Can you work these out from the model? Positions are in its coordinate system, mm. Face numbers are marked on the shaded views. Coordinates: 2 decimals unless noted, no trailing zeros. Write each loop counter-clockwise with the first axis right and the second up, starting at its lowest first coordinate (ties: lowest second). Pieces come first, ordered by that corner, then holes. Notation, with made-up numbers: (62, 71.5) -> (100, 71.5) arc R12 cw to (100, 80.5) -> close; hole circle Ø7 at (4, -26.75). An arc over 180 degrees is marked (long way). Use one line per item in the form item = value.
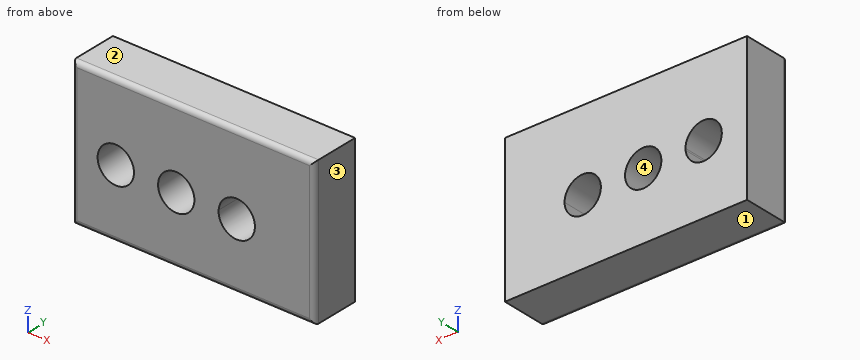
```python
from build123d import *

# Parameters (mm, degrees)
F0_W     = 254
F0_H     = 152.4
F1_DEPTH = 50.8
F3_DEPTH = 123.19
F4_R     = 5.08


with BuildPart() as f1:
    # F0 (on Front) → F1 (new body)
    with BuildSketch(Plane.XZ):
        with Locations((30.619834, 5.991532)):
            Rectangle(F0_W, F0_H)
    extrude(amount=F1_DEPTH)

    # F2 (on face) → F3 (cut)
    with BuildSketch(Plane.XZ.offset(50.8)):
        with BuildLine():
            ThreePointArc((-6.468596, 0), (12.581404, -19.05), (31.631404, 0))
            ThreePointArc((31.631404, 0), (12.581404, 19.05), (-6.468596, 0))
        make_face()
        with BuildLine():
            ThreePointArc((-31.782277, 1.811433), (-69.860685, 2.718177), (-31.868596, 0))
            ThreePointArc((-31.868596, 0), (-31.803869, 0.904689), (-31.782277, 1.811433))
        make_face()
        with BuildLine():
            ThreePointArc((95.098651, -1.116608), (76.607195, 17.925202), (57.031404, 0))
            ThreePointArc((57.031404, 0), (75.490107, -20.158418), (95.098651, -1.116608))
        make_face()
    extrude(amount=-F3_DEPTH, mode=Mode.SUBTRACT)

    # F4
    f4_edges = [f1.edges().sort_by_distance(p)[0] for p in [
        (30.619834, -50.8, -70.208468),
        (157.619834, -50.8, 5.991532),
        (30.619834, -50.8, 82.191532),
        (-96.380166, -50.8, 5.991532),
    ]]
    fillet(f4_edges, radius=F4_R)


solid = f1.part
```
Q1. Suppose I cut it at A-A (y = -35). Write out the boundary of the cut face in (x, z).
Return value:
outline = (-96.38, -70.21) -> (157.62, -70.21) -> (157.62, 82.19) -> (-96.38, 82.19) -> close; hole (-31.87, 0) arc R19.05 ccw to (-31.78, 1.81) arc R19.05 ccw (long way) to start; hole circle Ø38.1 at (12.58, 0); hole circle Ø38.1 at (76.05, -1.12)
Q2. If I drill on line 1 (X direction, y = -46, z = 13.5); line 2 (Z direction, x = 69, y = -15); line 3 (X direction, y = -46, z = -32), over which ranges is the centre line in solid material (lowest first)? Write a range as from..to.
Return value:
line_1 = -96.37..-65.87, -35.79..-0.86, 26.02..63.83, 88.27..157.61
line_2 = -70.21..-18.81, 16.58..82.19
line_3 = -96.37..157.61
Q3. Thinking about a two-plate mould opening in Z: for the marked faces 1, 2, 3 and 4, which applies, released by +Z, released by -Z, zero draft, split by the parting line, or undercut?
Return value:
face_1 = released by -Z
face_2 = released by +Z
face_3 = zero draft
face_4 = undercut
Q4. Suppose I cut it at D-D (x = 86). Write out the boundary of the cut face in (y, z).
Return value:
outline = (-50.8, -65.13) arc R5.08 ccw to (-45.72, -70.21) -> (0, -70.21) -> (0, -17.36) -> (-50.8, -17.36) -> close; (-50.8, 15.13) -> (0, 15.13) -> (0, 82.19) -> (-45.72, 82.19) arc R5.08 ccw to (-50.8, 77.11) -> close
Q5. Suppose I cut it at C-C (z = 13). Write out the boundary of the cut face in (x, y).
Return value:
outline = (-96.38, -45.72) arc R5.08 ccw to (-91.3, -50.8) -> (-66.25, -50.8) -> (-66.25, 0) -> (-96.38, 0) -> close; (-35.41, -50.8) -> (-1.34, -50.8) -> (-1.34, 0) -> (-35.41, 0) -> close; (26.51, -50.8) -> (63.26, -50.8) -> (63.26, 0) -> (26.51, 0) -> close; (88.84, -50.8) -> (152.54, -50.8) arc R5.08 ccw to (157.62, -45.72) -> (157.62, 0) -> (88.84, 0) -> close
Q6. Suppose I cut it at B-B (x = 8). Write out the boundary of the cut face in (y, z).
Return value:
outline = (-50.8, -65.13) arc R5.08 ccw to (-45.72, -70.21) -> (0, -70.21) -> (0, -18.49) -> (-50.8, -18.49) -> close; (-50.8, 18.49) -> (0, 18.49) -> (0, 82.19) -> (-45.72, 82.19) arc R5.08 ccw to (-50.8, 77.11) -> close
Q7. Will this pin go through, and if not, where does the flat tip stop? pin 1 (2 mm diameter, centred on x = 85.5, z = -46, fed in from +Y).
Return value:
pin_1 = 0
